```python
from build123d import *

# Parameters (mm, degrees)
F0_W     = 16.7
F0_H     = 24.2
F0_R     = 1.5
F0_R_2   = 3
F1_DEPTH = 2
F4_DEPTH = 5


with BuildPart() as f1:
    # F0 (on Top) → F1 (new body)
    with BuildSketch(Plane.XY):
        Rectangle(F0_W, F0_H)
        with Locations((-3, -9.1)):
            Circle(F0_R, mode=Mode.SUBTRACT)
        with Locations((3, -9.1)):
            Circle(F0_R, mode=Mode.SUBTRACT)
        with Locations((-3, 9.1)):
            Circle(F0_R, mode=Mode.SUBTRACT)
        Circle(F0_R_2, mode=Mode.SUBTRACT)
        with Locations((3, 9.1)):
            Circle(F0_R, mode=Mode.SUBTRACT)
    extrude(amount=F1_DEPTH)

    # F3 (on Right) → F4 (join, symmetric)
    with BuildSketch(Plane.YZ):
        Polygon((-4.1, 0), (-6.64, 0), (-6, -3.9), (-5, -3.9), (-3.85, -3.4), (-4.1, -2.9), align=None)
        Polygon((6.64, 0), (4.1, 0), (4.1, -2.9), (3.85, -3.4), (5, -3.9), (6, -3.9), align=None)
    extrude(amount=F4_DEPTH, both=True)


solid = f1.part
```
Here's how the part is built. I have some questions about the finished solid (model axes, mm). A direction names the side the tool comes from. Coordinates: 2 decimals unless noted, no trailing zeros. Loops run counter-clockwise (first coordinate to the right, second up) from the corner with the lowest first, then second, coordinate; pieces in that order, holes last. Notation, with made-up numbers: (59, -39) -> (117, -39) arc R13 cw to (117, -16) -> close; hole circle Ø3 at (75.25, 80.5). An arc over 180 degrees is marked (long way). Return JSON: item names as keys, results as strings.
1) If we section it at A-A, the plane y = 9.1: Write out the boundary of the cut face in (x, z), then the cut area to 3 significant figures.
Results below:
{"outline": "(-8.35, 0) -> (-4.5, 0) -> (-4.5, 2) -> (-8.35, 2) -> close; (-1.5, 0) -> (1.5, 0) -> (1.5, 2) -> (-1.5, 2) -> close; (4.5, 0) -> (8.35, 0) -> (8.35, 2) -> (4.5, 2) -> close", "area": "21.4 mm²"}
2) I need wall thicknesses on line 1 (X direction, y = -10, z = 0.4); line 2 (Z direction, x = -5.25, y = 2.5); line 3 (Y direction, x = 2, z = 0.3). Which ranges of each line are inside material? Lowest first, please. Write a range as from..to.
Results below:
{"line 1": "-8.35..-4.2, -1.8..1.8, 4.2..8.35", "line 2": "0..2", "line 3": "-12.1..-10.22, -7.98..-2.24, 2.24..7.98, 10.22..12.1"}
3) If we section it at B-B, the plane z = -0.85: Write out the boundary of the cut face in (x, y), then the cut area to 3 significant figures.
Results below:
{"outline": "(-5, -6.5) -> (5, -6.5) -> (5, -4.1) -> (-5, -4.1) -> close; (-5, 4.1) -> (5, 4.1) -> (5, 6.5) -> (-5, 6.5) -> close", "area": "48.0 mm²"}
4) If we section it at D-D, the plane y = 5.25: Write out the boundary of the cut face in (x, z).
Results below:
{"outline": "(-8.35, 0) -> (-5, 0) -> (-5, -3.9) -> (5, -3.9) -> (5, 0) -> (8.35, 0) -> (8.35, 2) -> (-8.35, 2) -> close"}
5) For faces 4 (the face through (-5, -5, -2)), 5 (the face through (5, -5, -2)), 6 (the face through (0, -4.1, -1)), which set-ups out of +Z, -Z, +X, -X, +Y, -Y let a thin tool reach every point of the face, with its end or its side?
Results below:
{"face 4": "-Z, -X, +Y, -Y", "face 5": "-Z, +X, +Y, -Y", "face 6": "+X, -X"}
6) Thinking about a two-plate mould opening in X: for faces 1 (the face through (-2.194, 10.365, 0.986)), 2 (the face through (8.35, 0, 1)), 3 (the face through (-0.07, -6.324, -1.923)), which applies, +X half, -X half, draft (parallel to the pull), parting line (faces both ways), or undercut?
Results below:
{"face 1": "undercut", "face 2": "+X half", "face 3": "draft"}
7) If we section it at C-C, the plane y = 0: Write out the boundary of the cut face in (x, z).
Results below:
{"outline": "(-8.35, 0) -> (-3, 0) -> (-3, 2) -> (-8.35, 2) -> close; (3, 0) -> (8.35, 0) -> (8.35, 2) -> (3, 2) -> close"}
8) Will these pins go through, and if not, where does the flat tip stop? pin 1 (1.5 mm diameter, centred on y = 7.5, z = -1.5, fed in from +X); pin 2 (0.9 mm diameter, centred on x = 0, z = -2, fed in from -Y); pin 3 (1.4 mm diameter, centred on x = -0.5, z = -1, fed in from +Y); pin 4 (3.5 mm diameter, centred on x = 3, y = 9.1, fed in from -Z).
Results below:
{"pin 1": "through", "pin 2": "y = -6.39", "pin 3": "y = 6.59", "pin 4": "z = 0"}
